Can you work these out from the model? Positions are in its coordinate system, mm. Coordinates: 2 decimals unless noted, no trailing zeros. Write each loop counter-clockwise with the first axis right and the second up, starting at its lowest first coordinate (ties: lowest second). Pieces come first, ordered by that corner, then holes. Notation, with made-up numbers: (18, -31) -> (30, -31) arc R12 cw to (30, -18) -> close; hole circle Ø7 at (-7.75, -27). An arc over 180 degrees is marked (long way). Use one line per item in the form item = value.
```python
from build123d import *

# Parameters (mm, degrees)
SKIZZE16_R                      = 2.5
AUFSATZ_LINEAR_AUSTRAGEN1_DEPTH = 4


with BuildPart() as part:
    # Skizze16 → Aufsatz-Linear austragen1 (new body)
    with BuildSketch(Plane.XZ.offset(5)):
        with BuildLine():
            Line((5.975062847, -6.5), (5.975062847, -14))
            ThreePointArc((5.975062847, -14), (0, -19.975062847), (-5.975062847, -14))
            Line((-5.975062847, -14), (-5.975062847, -6.5))
            ThreePointArc((-5.975062847, -6.5), (0, -0.524937153), (5.975062847, -6.5))
        make_face()
        with Locations(Location((0, -14, 0), (0, 0, 270))):
            Circle(SKIZZE16_R, mode=Mode.SUBTRACT)
        with Locations(Location((0, -6.5, 0), (0, 0, 270))):
            Circle(SKIZZE16_R, mode=Mode.SUBTRACT)
    extrude(amount=AUFSATZ_LINEAR_AUSTRAGEN1_DEPTH)


solid = part.part
```
Q1. Thinking about a two-plate mould opening in Z: for faces 1 (the flat face through (0, -5, -10)), 2 (the cylindrical face through (0.131, -6.972, -19.974)), 3 (the cylindrical face through (0.751, -6.972, -8.885)), which applies, released by +Z, released by -Z, zero draft, split by the parting line, or undercut?
Return value:
face_1 = zero draft
face_2 = released by -Z
face_3 = undercut
Q2. Suppose I cut it at A-A (x = 0). Write out the boundary of the cut face in (y, z).
Return value:
outline = (-9, -19.98) -> (-5, -19.98) -> (-5, -16.5) -> (-9, -16.5) -> close; (-9, -11.5) -> (-5, -11.5) -> (-5, -9) -> (-9, -9) -> close; (-9, -4) -> (-5, -4) -> (-5, -0.52) -> (-9, -0.52) -> close
Q3. If I drill on line 1 (X direction, y = -8.05, z = -14); line 2 (Z direction, x = -2, y = -6.95); line 3 (Z direction, x = -1.25, y = -8.15), over which ranges is the centre line in solid material (lowest first)? Write a range as from..to.
Return value:
line_1 = -5.98..-2.5, 2.5..5.98
line_2 = -19.63..-15.5, -12.5..-8, -5..-0.87
line_3 = -19.84..-16.17, -11.83..-8.67, -4.33..-0.66
Q4. Will these pins go through, and if not, where does the flat tip stop? pin 1 (4.5 mm diameter, centred on x = 0, z = -6.5, fed in from +Y); pin 2 (1 mm diameter, centred on x = 3.5, y = -8, fed in from +Z); pin 3 (1.5 mm diameter, centred on x = 3, y = -7, fed in from -Z).
Return value:
pin_1 = through
pin_2 = -1.33
pin_3 = -19.54
Q5. Suppose I cut it at D-D (z = -5.75). Write out the boundary of the cut face in (x, y), then the cut area to 3 significant figures.
Return value:
outline = (-5.93, -9) -> (-2.38, -9) -> (-2.38, -5) -> (-5.93, -5) -> close; (2.38, -9) -> (5.93, -9) -> (5.93, -5) -> (2.38, -5) -> close
area = 28.3 mm2
Q6. Suppose I cut it at C-C (y = -7). Write out the boundary of the cut face in (x, z), then the cut area to 3 significant figures.
Return value:
outline = (-5.98, -14) arc R5.98 ccw to (5.98, -14) -> (5.98, -6.5) arc R5.98 ccw to (-5.98, -6.5) -> close; hole circle Ø5 at (0, -14); hole circle Ø5 at (0, -6.5)
area = 163 mm2
Q7. Suppose I cut it at B-B (z = -13.5). Write out the boundary of the cut face in (x, y), then the cut area to 3 significant figures.
Return value:
outline = (-5.98, -9) -> (-2.45, -9) -> (-2.45, -5) -> (-5.98, -5) -> close; (2.45, -9) -> (5.98, -9) -> (5.98, -5) -> (2.45, -5) -> close
area = 28.2 mm2
